```python
from build123d import *

# Parameters (mm, degrees)
BOSS_EXTRUDE1_DEPTH     = 12.7
CUT_EXTRUDE1_REACH      = 36.341
SKETCH2_R               = 5
BOSS_EXTRUDE3_OUTLINE_R = 12.5
BOSS_EXTRUDE3_DEPTH     = 20.5


# Read off the part's stored shape, not the designer's step: Boss-Extrude3
with BuildPart() as part:
    # Sketch1 → Boss-Extrude1 (new body)
    with BuildSketch(Plane(origin=(0, 0, 0), x_dir=(-1, 0, 0), z_dir=(0, 0, -1))):
        Polygon((22.52557458, -1.736588639), (22.52557458, 0.194536921), (19.229808022, 0.93665661), (15.128723263, 11.851737372), (17.063649078, 14.621011813), (15.786423571, 16.069438867), (12.890863827, 14.329165151), (2.313040546, 19.235032954), (1.719665356, 22.560799741), (-0.211460204, 22.560799741), (-0.98374926, 19.271971918), (-11.902473648, 15.180597821), (-14.673902719, 17.112436257), (-16.073066924, 15.781427071), (-14.308800518, 12.900423272), (-19.236913758, 2.332945609), (-22.560976284, 1.730096406), (-22.560976284, -0.201029153), (-19.275488766, -0.987407309), (-15.174404006, -11.902488071), (-17.112216048, -14.669743631), (-15.788139908, -16.075470597), (-12.910837913, -14.305173427), (-2.333014633, -19.21104123), (-1.727718406, -22.534659035), (0.203407153, -22.534659035), (0.978499423, -19.246490729), (11.89722381, -15.155116632), (14.659649692, -17.099807376), (16.072878525, -15.783741196), (14.276312796, -12.922767512), (19.204426036, -2.355289849), align=None)
    extrude(amount=-BOSS_EXTRUDE1_DEPTH)

    # Sketch2 → Cut-Extrude1 (cut, up to next)
    with BuildSketch(Plane(origin=(0, 0, 0), x_dir=(-1, 0, 0), z_dir=(0, 0, -1)), mode=Mode.PRIVATE) as cut_extrude1_sk1:
        with Locations((-0.019773646, -0.00956531)):
            Circle(SKETCH2_R)
    cut_extrude1_tool1 = extrude(cut_extrude1_sk1.sketch, amount=-CUT_EXTRUDE1_REACH, mode=Mode.PRIVATE) & part.part
    add(cut_extrude1_tool1.solids().sort_by_distance((0.019774, -0.009565, 0))[0], mode=Mode.SUBTRACT)

    # Boss-Extrude3 outline → Boss-Extrude3 (add)
    with BuildSketch(Plane(origin=(0, 0, 0), x_dir=(-1, 0, 0), z_dir=(0, 0, -1))):
        Circle(BOSS_EXTRUDE3_OUTLINE_R)
        with BuildLine():
            ThreePointArc((2.167436153, -4.505798544), (-4.520800394, -2.186893539), (-2.187209799, 4.496233234))
            ThreePointArc((-2.187209799, 4.496233234), (4.501026748, 2.177328229), (2.167436153, -4.505798544))
        make_face(mode=Mode.SUBTRACT)
    extrude(amount=BOSS_EXTRUDE3_DEPTH)


solid = part.part
```
CAD build for the part. Positions are in the model's coordinates, mm. A direction names the side the tool comes from. Round coordinates to 2 decimals unless told otherwise and drop trailing zeros. Write each loop counter-clockwise with the first axis right and the second up, starting at its lowest first coordinate (ties: lowest second). Pieces come first, ordered by that corner, then holes. Notation, with made-up numbers: (-38, -5.5) - (-32, -5.5) arc R12 cw to (-32, 7.5) - close; hole circle Ø1 at (87.5, 81). An arc over 180 degrees is marked (long way). Return JSON: item names as keys, results as strings. Group by question number.
Item 1: Band-saw the part on A-A on z = -12. List the corners of the cut face in (x, y), plus the area to 3 significant figures.
Item 2: Band-saw the part on C-C on x = 9. List the corners of the cut face in (y, z), plus the area to 3 significant figures.
Item 3: Probe probe 1 along Y at (x, z) = (-4, -8); probe 2 along X at (y, z) = (-2, -8); probe 3 along Z at (x, y) = (12, 9). List the from-to ranges inside material, lowest first.
Item 4: Mould opens along X. For faces 4 (the face through (-1, 22.561, 6)), 5 (the face through (-15.36, -16.45, 6.26)), 6 (the face through (-7.676, 16.748, 6.261)) say: +X half, -X half, draft (parallel to the pull), parting line (faces both ways), or undercut.
Item 5: 3-axis set-ups, long thin cutter, end or side, ignore diameter. For faces 1 (the face through (-14.36, 15.21, 6.26)), 2 (the face through (-11.923, 3.755, -10.106)), 3 (the face through (17.254, -6.369, 6.261)): which of +Z, -Z, +X, -X, +Y, -Y reach the whole face in a straight line?
Item 6: Flat gauge pins, fed straight in: pin 1 Ø1 at (y, z) = (16, 2.5) entering from -X; pin 2 Ø5 at (y, z) = (1.5, -12) entering from +X; pin 3 Ø3.5 at (x, y) = (-1, 2) entering from -Z; pin 4 Ø1 at (y, z) = (-6, -9) entering from -X (3 decimals). Where does each tip first touch, or does it go through?
Item 7: Band-saw the part on B-B on y = -7.5. List the corners of the cut face in (x, z).
Resolved:
{
 "1": {"outline": "circle Ø25 at (0, 0); hole (-2.17, -4.51) arc R5 ccw to (2.19, 4.5) arc R5 ccw to start", "area": "412 mm²"},
 "2": {"outline": "(-16.12, 0) - (-8.67, 0) - (-8.67, -20.5) - (8.67, -20.5) - (8.67, 0) - (16.27, 0) - (16.27, 12.7) - (-16.12, 12.7) - close", "area": "767 mm²"},
 "3": {"probe 1": "y = -11.84 to -3, 3 to 11.84", "probe 2": "x = -12.34 to -4.58, 4.61 to 12.34", "probe 3": "z = 0 to 12.7"},
 "4": {"face 4": "draft", "face 5": "-X half", "face 6": "undercut"},
 "5": {"face 1": "+Z, -Z, +Y", "face 2": "-Z", "face 3": "+Z, -Z, +X"},
 "6": {"pin 1": "stops at x = -16.29", "pin 2": "stops at x = 12.5", "pin 3": "passes through", "pin 4": "stops at x = -11.225"},
 "7": {"outline": "(-16.81, 0) - (-10, 0) - (-10, -20.5) - (10, -20.5) - (10, 0) - (16.83, 0) - (16.83, 12.7) - (-16.81, 12.7) - close"}
}
